from build123d import *

# Parameters (mm, degrees)
BOSS_EXTRUDE2_DEPTH = 100
CUT_EXTRUDE1_DEPTH  = 121.933866224
BOSS_EXTRUDE6_DEPTH = 15
BOSS_EXTRUDE8_START = -15
BOSS_EXTRUDE8_DEPTH = 15
SKETCH10_R          = 15
CUT_EXTRUDE2_DEPTH  = 151.934588481


with BuildPart() as part:
    # Sketch2 → Boss-Extrude2 (new body)
    with BuildSketch(Plane.XY):
        Polygon((65, 0), (45, 20), (-65, 20), (-65, 0), align=None)
    extrude(amount=-BOSS_EXTRUDE2_DEPTH)

    # Sketch3 → Cut-Extrude1 (cut, through all)
    with BuildSketch(Plane(origin=(0, 20, 0), x_dir=(1, 0, 0), z_dir=(0, 1, 0))):
        with BuildLine():
            Line((65, 70), (15, 70))
            ThreePointArc((15, 70), (-5, 50), (15, 30))
            Line((15, 30), (65, 30))
            Line((65, 30), (65, 70))
        make_face()
    extrude(amount=-CUT_EXTRUDE1_DEPTH, mode=Mode.SUBTRACT)

    # Sketch4 → Boss-Extrude6 (add)
    with BuildSketch(Plane.XY):
        with BuildLine():
            Line((-65, 20), (-65, 72.98579059))
            ThreePointArc((-65, 72.98579059), (-47.439143931, 91.99502078), (-23.607384696, 81.906326611))
            Line((-23.607384696, 81.906326611), (15, 20))
            Line((15, 20), (-65, 20))
        make_face()
    extrude(amount=-BOSS_EXTRUDE6_DEPTH)

    # Sketch9 → Boss-Extrude8 (add)
    with BuildSketch(Plane(origin=(0, 0, -100), x_dir=(-1, 0, 0), z_dir=(0, 0, -1)).offset(BOSS_EXTRUDE8_START)):
        with BuildLine():
            Line((-15, 20), (23.607384696, 81.906326611))
            ThreePointArc((23.607384696, 81.906326611), (47.439143931, 91.99502078), (65, 72.98579059))
            Line((65, 72.98579059), (65, 20))
            Line((65, 20), (-15, 20))
        make_face()
    extrude(amount=BOSS_EXTRUDE8_DEPTH)

    # Sketch10 → Cut-Extrude2 (cut, through all)
    with BuildSketch(Plane.XY):
        with Locations((-42.698989831, 70)):
            Circle(SKETCH10_R)
    extrude(amount=-CUT_EXTRUDE2_DEPTH, mode=Mode.SUBTRACT)


solid = part.part
Verification items for the finished model (mm, model axes). A direction names the side the tool comes from. Give positions to 0.01 mm unless a question says otherwise; leave off trailing zeros. Loops run counter-clockwise (first coordinate to the right, second up) from the corner with the lowest first, then second, coordinate; pieces in that order, holes last.
1) Sectioned sample at B-B, the plane x = 56.5. Enter the section's corners in (y, z), then the cut area to 3 significant figures.
2) Draft check along Z on faces 1 (the flat face through (35, 10, -70)), 2 (the cylindrical face through (-35.78, 56.69, -7.4)), 3 (the flat face through (-14, 26, 0)). Enter one of: pulls with the +Z half, pulls with the -Z half, needs draft (parallel to the pull), parting line crosses it, or undercut.
3) Depth check by flat-ended pin: pin 1 Ø5 at (x, z) = (-31, -39) entering from -Y; pin 2 Ø1 at (x, z) = (18.5, -17) entering from +Y. Enter the tip coordinate at first touch or a pass-through.
4) Sectioned sample at D-D, the plane z = -50. Enter the section's corners in (x, y).
5) Sectioned sample at C-C, the plane y = 70. Enter the section's corners in (x, z), then the cut area to 3 significant figures.
6) Set-up check for faces 4 (the flat face through (34, 10, -30)), 5 (the flat face through (-4.574, 51.387, -7.395)), 6 (the flat face through (-33, 49, -15)): record each of +Z, -Z, +X, -X, +Y, -Y from which the full face is reachable in a straight line by a thin tool's end or side.
7) Sectioned sample at A-A, the plane y = 17.5. Enter the section's corners in (x, z), then the cut area to 3 significant figures.
8) Thickness scan on line 1 along Z through (x, y) = (23.5, 14); line 2 along Y through (x, z) = (16, -28.5); line 3 along Z through (x, y) = (-46, 51.5). Record the ranges inside material, lowest first.
Answers:
1. outline: (0, -100) - (8.5, -100) - (8.5, -70) - (0, -70) - close; (0, -30) - (8.5, -30) - (8.5, 0) - (0, 0) - close
1. area: 510 mm2
2. face 1: undercut
2. face 2: needs draft
2. face 3: pulls with the +Z half
3. pin 1: stops at y = 0
3. pin 2: stops at y = 20
4. outline: (-65, 0) - (-5, 0) - (-5, 20) - (-65, 20) - close
5. outline: (-65, -100) - (-57.7, -100) - (-57.7, -85) - (-65, -85) - close; (-65, -15) - (-57.7, -15) - (-57.7, 0) - (-65, 0) - close; (-27.7, -100) - (-16.18, -100) - (-16.18, -85) - (-27.7, -85) - close; (-27.7, -15) - (-16.18, -15) - (-16.18, 0) - (-27.7, 0) - close
5. area: 565 mm2
6. face 4: +X, +Y, -Y
6. face 5: +Z, -Z, +X, +Y
6. face 6: +X, -X, +Y
7. outline: (-65, -100) - (47.5, -100) - (47.5, -70) - (15, -70) arc R20 cw to (15, -30) - (47.5, -30) - (47.5, 0) - (-65, 0) - close
7. area: 9,320 mm2
8. line 1: z = -100 to -70, -30 to 0
8. line 2: y = 0 to 20
8. line 3: z = -100 to -85, -15 to 0
